Read the model definition and answer for the solid it produces. Units are mm, in the model's axes. Face numbers are marked on the shaded views. A direction names the side the tool comes from. Coordinates: 2 decimals unless noted, no trailing zeros. Loops run counter-clockwise (first coordinate to the right, second up) from the corner with the lowest first, then second, coordinate; pieces in that order, holes last.
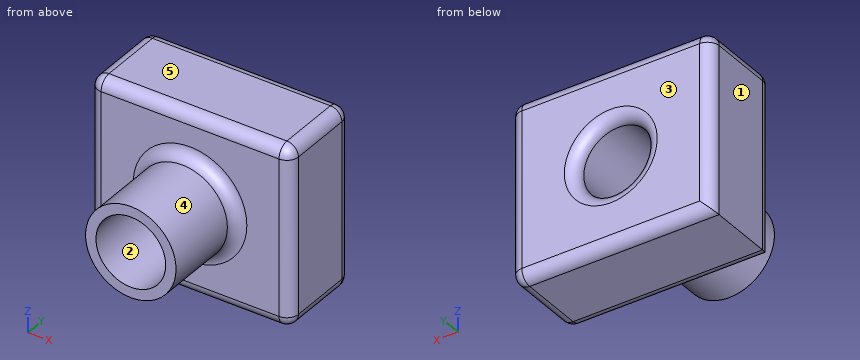
from build123d import *

# Parameters (mm, degrees)
F0_W     = 88.3796066046
F0_H     = 78.8212642074
F1_DEPTH = 38.1
F2_R     = 19.8886852244
F3_DEPTH = 76.2
F4_R     = 15.3300862408
F5_DEPTH = 101.6
F6_R     = 5.08


with BuildPart() as f1:
    # F0 (on Front) → F1 (new body)
    with BuildSketch(Plane.XZ):
        Rectangle(F0_W, F0_H)
    extrude(amount=F1_DEPTH)

    # F2 (on Front) → F3 (join)
    with BuildSketch(Plane.XZ):
        Circle(F2_R)
    extrude(amount=F3_DEPTH)

    # F4 (on face) → F5 (cut)
    with BuildSketch(Plane.XZ.offset(76.2)):
        Circle(F4_R)
    extrude(amount=-F5_DEPTH, mode=Mode.SUBTRACT)

    # F6
    f6_edges = [f1.edges().sort_by_distance(p)[0] for p in [
        (-44.189803, -19.05, 39.410632),
        (0, 0, 39.410632),
        (0, -38.1, 39.410632),
        (44.189803, -38.1, 0),
        (-44.189803, -38.1, 0),
        (0, -38.1, -39.410632),
        (-19.888685, -38.1, 0),
        (44.189803, -19.05, -39.410632),
        (44.189803, -19.05, 39.410632),
        (44.189803, 0, 0),
        (-44.189803, 0, 0),
        (0, 0, -39.410632),
        (-15.330086, 0, 0),
    ]]
    fillet(f6_edges, radius=F6_R)


solid = f1.part
Q1. A cutting plane is placed at B-B (x = 0). Give the vertices of the cut face in (y, z), then the cut area to 3 significant figures.
Findings below:
outline: (-76.2, -19.89) - (-43.18, -19.89) arc R5.08 cw to (-38.1, -24.97) - (-38.1, -34.33) arc R5.08 ccw to (-33.02, -39.41) - (-5.08, -39.41) arc R5.08 ccw to (0, -34.33) - (0, -20.41) arc R5.08 ccw to (-5.08, -15.33) - (-76.2, -15.33) - close; (-76.2, 15.33) - (-5.08, 15.33) arc R5.08 ccw to (0, 20.41) - (0, 34.33) arc R5.08 ccw to (-5.08, 39.41) - (-33.02, 39.41) arc R5.08 ccw to (-38.1, 34.33) - (-38.1, 24.97) arc R5.08 cw to (-43.18, 19.89) - (-76.2, 19.89) - close
area: 2,160 mm2
Q2. Flat-ended cylindrical pins translate along their axes: pin 1 Ø2 at (x, y) = (6, -64.5) entering from +Z; pin 2 Ø6 at (y, z) = (-61.5, 9) entering from +X; pin 3 Ø1.5 at (x, y) = (-7, -50) entering from +Z; pin 4 Ø12 at (x, z) = (-3.5, 3) entering from -Y. Find the tip coordinate at first contact, or state that the pin passes through.
Findings below:
pin 1: stops at z = 19.25
pin 2: stops at x = 18.96
pin 3: stops at z = 18.88
pin 4: passes through
Q3. A cutting plane is placed at C-C (y = -22). Give the vertices of the cut face in (x, z).
Findings below:
outline: (-44.19, -39.41) - (39.11, -39.41) arc R5.08 ccw to (44.19, -34.33) - (44.19, 34.33) arc R5.08 ccw to (39.11, 39.41) - (-39.11, 39.41) arc R5.08 ccw to (-44.19, 34.33) - close; hole circle Ø30.66 at (0, 0)
Q4. A cutting plane is placed at D-D (z = 27). Give the vertices of the cut face in (x, y).
Findings below:
outline: (-44.19, -33.02) arc R5.08 ccw to (-39.11, -38.1) - (39.11, -38.1) arc R5.08 ccw to (44.19, -33.02) - (44.19, -5.08) arc R5.08 ccw to (39.11, 0) - (-39.11, 0) arc R5.08 ccw to (-44.19, -5.08) - close
Q5. A cutting plane is placed at A-A (z = 0). Give the vertices of the cut face in (x, y).
Findings below:
outline: (-44.19, -33.02) arc R5.08 ccw to (-39.11, -38.1) - (-24.97, -38.1) arc R5.08 cw to (-19.89, -43.18) - (-19.89, -76.2) - (-15.33, -76.2) - (-15.33, -5.08) arc R5.08 ccw to (-20.41, 0) - (-39.11, 0) arc R5.08 ccw to (-44.19, -5.08) - close; (15.33, -76.2) - (19.89, -76.2) - (19.89, -43.18) arc R5.08 cw to (24.97, -38.1) - (39.11, -38.1) arc R5.08 ccw to (44.19, -33.02) - (44.19, -5.08) arc R5.08 ccw to (39.11, 0) - (20.41, 0) arc R5.08 ccw to (15.33, -5.08) - close
Q6. Determine the mould class of the marked faces 1, 2 and 3 for opening direction X: +X half, -X half, draft (parallel to the pull), parting line (faces both ways), or undercut.
Findings below:
face 1: -X half
face 2: undercut
face 3: draft
Q7. Straight lines are drawn through the part: probe 1 along X at (y, z) = (-51.5, -0.5); probe 2 along Z at (x, y) = (0, -48); probe 3 along Y at (x, z) = (2, 25.5). For each, find the intervals that lie inside material, in ascending order.
Findings below:
probe 1: x = -19.88 to -15.32, 15.32 to 19.88
probe 2: z = -19.89 to -15.33, 15.33 to 19.89
probe 3: y = -38.1 to 0
Q8. Which of the six approach directions +Z, -Z, +X, -X, +Y, -Y give full straight-line access (tool end or side, diameter ignored) to the marked faces 4 and 5?
Findings below:
face 4: -Y
face 5: +Z, +X, -X, +Y, -Y
